Build history of the part. All positions in model axes, mm. A direction names the side the tool comes from. Give positions to 0.01 mm unless a question says otherwise; leave off trailing zeros. Loops run counter-clockwise (first coordinate to the right, second up) from the corner with the lowest first, then second, coordinate; pieces in that order, holes last.
1) Wall check: line 1 (X direction, y = 501, z = -64); line 2 (Z direction, x = 63, y = 761). Give the ranges that are in metal, low to high.
2) Band-saw the part on C-C on z = -43. List the corners of the cut face in (x, y).
3) Band-saw the part on A-A on y = 884. List the corners of the cut face in (x, z), then the cut area to 3 significant figures.
4) 3-axis set-ups, long thin cutter, end or side, ignore diameter. For faces 1 (the flat face through (25.4, 501, -50)), 2 (the flat face through (38, 501, 0)): which of +Z, -Z, +X, -X, +Y, -Y reach the whole face in a straight line?
5) Flat gauge pins, fed straight in: P1, Ø12, axis at y = 418.5, z = -54.5, coming from the +X side; P2, Ø3, axis at x = 37, y = 278.5, coming from the -Z side. Where does each tip first touch, or does it go through?
6) Band-saw the part on B-B on x = 57.5. List the corners of the cut face in (y, z), then the cut area to 3 significant figures.
Autodesk Inventor part; units mm, degrees
ref_plane "YZ Plane" through (0, 0, 0) normal (1, 0, 0) x (0, 1, 0)
ref_plane "XZ Plane" through (0, 0, 0) normal (0, 1, 0) x (-1, 0, 0)
ref_plane "XY Plane" through (0, 0, 0) normal (0, 0, 1) x (1, 0, 0)
sketch "Sketch1" plane through (0, 0, 0) normal (0, 1, 0) x (-1, 0, 0)
  line L0 (0, 0) -> (-25.4, 0)
  line L1 (-25.4, 0) -> (-25.4, -25.4)
  line L2 (-25.4, -25.4) -> (0, -25.4)
  line L3 (0, -25.4) -> (0, 0)
  dimension "d0" = 25.4
  dimension "d1" = 25.4
extrude "Extrusion1" add sketch "Sketch1" along normal blind 1016
sketch "Sketch2" plane through (25.4, 0, 0) normal (1, 0, 0) x (0, 0, -1)
  line L0 (0, 0) -> (25.4, 0)
  line L1 (0, 1016) -> (25.4, 1016)
  line L2 (25.4, 1016) -> (25.4, 0)
  line L3 (25.4, 0) -> (0, 0)
  line L4 (0, 0) -> (0, 1016)
extrude "Extrusion2" add sketch "Sketch2" along normal blind 50.8
sketch "Sketch4" plane through (0, 0, -25.4) normal (0, 0, -1) x (-1, 0, 0)
  line L0 (0, 0) -> (-76.2, 0)
  line L1 (0, 0) -> (-25.4, 0)
  line L2 (-25.4, 0) -> (-25.4, 1016)
  line L3 (-25.4, 1016) -> (0, 1016)
  line L4 (0, 1016) -> (0, 0)
  dimension "d8" = 25.4
  dimension "d9" = 1016
extrude "Extrusion4" add sketch "Sketch4" along normal blind 50.8
properties part number "rev1 corners"
Findings below:
1. line 1: x = 0 to 25.4
1. line 2: z = -25.4 to 0
2. outline: (0, 0) - (25.4, 0) - (25.4, 1016) - (0, 1016) - close
3. outline: (0, -76.2) - (25.4, -76.2) - (25.4, -25.4) - (76.2, -25.4) - (76.2, 0) - (0, 0) - close
3. area: 3,230 mm2
4. face 1: -Z, +X, +Y, -Y
4. face 2: +Z, +X, -X, +Y, -Y
5. P1: stops at x = 25.4
5. P2: stops at z = -25.4
6. outline: (0, -25.4) - (1016, -25.4) - (1016, 0) - (0, 0) - close
6. area: 25,800 mm2
